The figure shows three views and two pictorial views of one solid part (mm, origin at its lowest corner). Answer the questions. A direction names the side the tool comes from. Coordinates: 2 decimals unless noted, no trailing zeros. Loops run counter-clockwise (first coordinate to the right, second up) from the corner with the lowest first, then second, coordinate; pieces in that order, holes last. Notation, with made-up numbers: M 84.25,32 L 128.25,32 A26 cw 128.25,69 Z; hole C 35,-25.5 d9. An arc over 180 degrees is marked long. Answer in a Markdown table with one row per item. Add a question column.
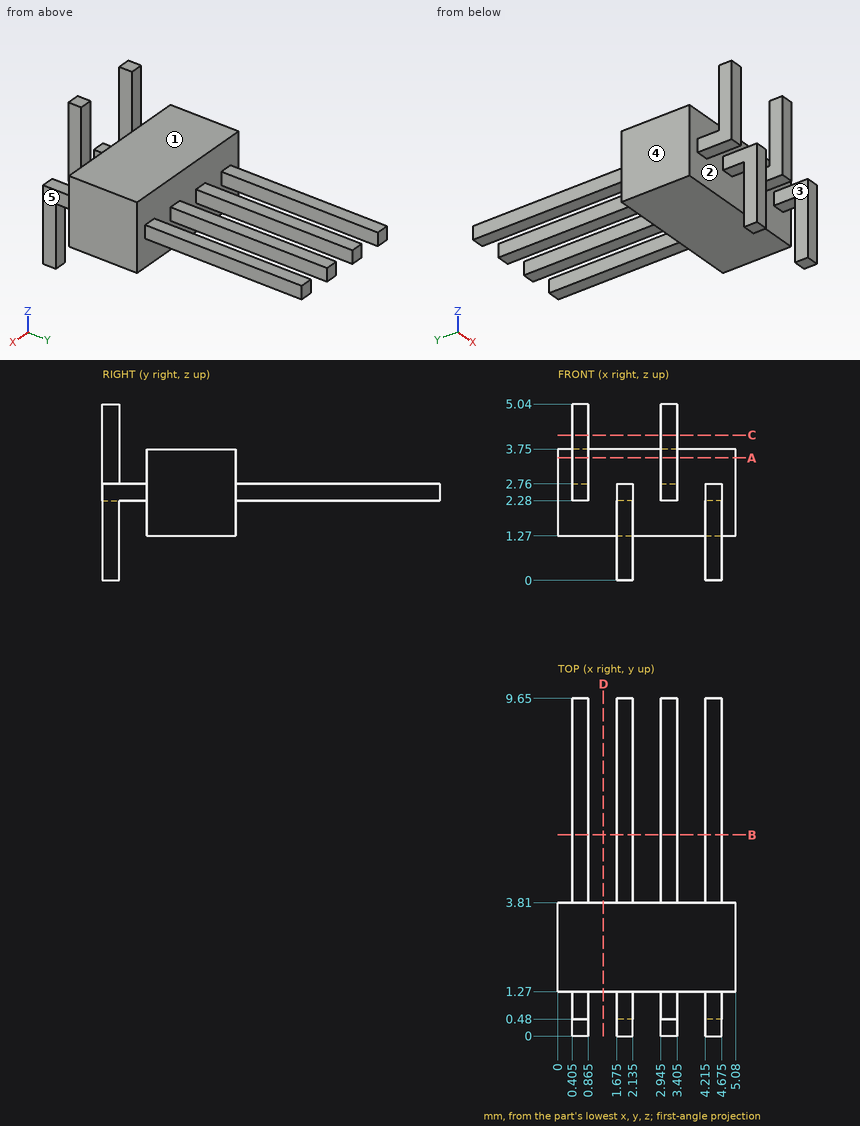
(1) A cutting plane is placed at A-A (z = 3.5). Give the vertices of the cut face in (x, y) (3 decimals).
(2) For the marked faces 3, 4 and 5, determine the directions among +Z, -Z, +X, -X, +Y, -Y from which every point of the face is accessible in a straight line to the end or side of a thin tool.
(3) Each of these flat-tipped pins is pushed along its axis until it touches: pin 1 (1 mm diameter, centred on x = 2, y = 6, fed in from +Z); pin 2 (1.5 mm diameter, centred on x = 3.5, z = 4, fed in from -Y); pin 3 (1 mm diameter, centred on y = 0.5, z = 1, fed in from -X) (3 decimals); pin 4 (0.5 mm diameter, centred on x = 0.5, y = 7, fed in from -Z). Where does it stop, or does it pass through?
(4) Straight lines are drawn through the part: line 1 (X direction, y = 1, z = 2.5) (3 decimals); line 2 (Z direction, x = 3.3, y = 6); line 3 (Y direction, x = 1.25, z = 2.1). For each, find the intervals that lie inside material, in ascending order.
(5) A cutting plane is placed at B-B (y = 5.75). Give the vertices of the cut face in (x, z) (3 decimals), plus the area to 3 significant figures.
(6) The mould has two halves that part along Y. Classify the marked faces 1 and 2: released by +Y, released by -Y, zero draft, split by the parting line, or undercut.
(7) A cutting plane is placed at C-C (z = 4.15). Give the vertices of the cut face in (x, y) (3 decimals).
(8) A cutting plane is placed at D-D (x = 1.3). Give the vertices of the cut face in (y, z), plus the area to 3 significant figures.
Solved:
| question | item | result |
|---|---|---|
| 1 | outline | M 0,1.27 L 5.08,1.27 L 5.08,3.81 L 0,3.81 Z; M 0.405,0 L 0.865,0 L 0.865,0.48 L 0.405,0.48 Z; M 2.945,0 L 3.405,0 L 3.405,0.48 L 2.945,0.48 Z |
| 2 | face 3 | +Z, -Z, -Y |
| 2 | face 4 | +Z, -Z, -X, +Y, -Y |
| 2 | face 5 | +Z, -Z, +X, -Y |
| 3 | pin 1 | stops at z = 2.76 |
| 3 | pin 2 | stops at y = 0 |
| 3 | pin 3 | stops at x = 1.675 |
| 3 | pin 4 | stops at z = 2.28 |
| 4 | line 1 | x = 0.405 to 0.865, 1.675 to 2.135, 2.945 to 3.405, 4.215 to 4.675 |
| 4 | line 2 | z = 2.28 to 2.76 |
| 4 | line 3 | y = 1.27 to 3.81 |
| 5 | outline | M 0.405,2.28 L 0.865,2.28 L 0.865,2.76 L 0.405,2.76 Z; M 1.675,2.28 L 2.135,2.28 L 2.135,2.76 L 1.675,2.76 Z; M 2.945,2.28 L 3.405,2.28 L 3.405,2.76 L 2.945,2.76 Z; M 4.215,2.28 L 4.675,2.28 L 4.675,2.76 L 4.215,2.76 Z |
| 5 | area | 0.883 mm² |
| 6 | face 1 | zero draft |
| 6 | face 2 | undercut |
| 7 | outline | M 0.405,0 L 0.865,0 L 0.865,0.48 L 0.405,0.48 Z; M 2.945,0 L 3.405,0 L 3.405,0.48 L 2.945,0.48 Z |
| 8 | outline | M 1.27,1.27 L 3.81,1.27 L 3.81,3.75 L 1.27,3.75 Z |
| 8 | area | 6.30 mm² |
